```python
from build123d import *

# Parameters (mm, degrees)
CUT_EXTRUDE_1_DEPTH = 125.373429638


with BuildPart() as part:
    # 草图1 → 旋转1 (revolve)
    with BuildSketch(Plane.XY, mode=Mode.PRIVATE) as revolve_1_sk:
        with BuildLine():
            Line((45, 37.5), (25, 37.5))
            ThreePointArc((25, 37.5), (0, 22.5), (-25, 37.5))
            Line((-25, 37.5), (-45, 37.5))
            ThreePointArc((-45, 37.5), (-71.516504294, 26.516504294), (-82.5, 0))
            Line((-82.5, 0), (82.5, 0))
            ThreePointArc((82.5, 0), (71.516504294, 26.516504294), (45, 37.5))
        make_face()
    revolve(revolve_1_sk.sketch.rotate(Axis((-82.5, 0, 0), (1, 0, 0)), 180), axis=Axis((-82.5, 0, 0), (1, 0, 0)))

    # 草图2 → 切除-拉伸1 (cut, through all)
    with BuildSketch(Plane(origin=(30, 0, 0), x_dir=(0, 0, -1), z_dir=(1, 0, 0))):
        with BuildLine():
            Line((10, 36.142080737), (10, 10))
            Line((10, 10), (36.142080737, 10))
            ThreePointArc((36.142080737, 10), (26.516504294, 26.516504294), (10, 36.142080737))
        make_face()
        with BuildLine():
            Line((-10, 10), (-36.142080737, 10))
            ThreePointArc((-36.142080737, 10), (-26.516504294, 26.516504294), (-10, 36.142080737))
            Line((-10, 36.142080737), (-10, 10))
        make_face()
        with BuildLine():
            Line((-10, -10), (-36.142080737, -10))
            ThreePointArc((-36.142080737, -10), (-26.516504294, -26.516504294), (-10, -36.142080737))
            Line((-10, -36.142080737), (-10, -10))
        make_face()
        with BuildLine():
            Line((10, -10), (36.142080737, -10))
            ThreePointArc((36.142080737, -10), (26.516504294, -26.516504294), (10, -36.142080737))
            Line((10, -36.142080737), (10, -10))
        make_face()
    cut_extrude_1 = extrude(amount=CUT_EXTRUDE_1_DEPTH, mode=Mode.SUBTRACT)

    # 镜向1: 切除-拉伸1 across plane
    add(cut_extrude_1.mirror(Plane(origin=(0, 0, 0), x_dir=(0, 0, 1), z_dir=(1, 0, 0))), mode=Mode.SUBTRACT)


solid = part.part
```
Geometry: final body of the model. Coordinates: model frame, mm. A direction names the side the tool comes from. Coordinates: 2 decimals unless noted, no trailing zeros. Order: outer loops, then holes, each group sorted by start corner. A loop starts at its lowest first (then second) coordinate and runs counter-clockwise, first axis right, second up. Notation, with made-up numbers: (-21.5, -9) -> (-7.5, -9) arc R29 ccw to (-7.5, 17) -> close; hole circle Ø9 at (4.5, 63). An arc over 180 degrees is marked (long way). Write item = value, one per line.
(1) Access query for faces 1 (the flat face through (-49, -10, 23)), 2 (the flat face through (-30, -20, -20)), 3 (the flat face through (30, 20, 20)), 4 (the flat face through (49, -20, -10)). Directions: +Z, -Z, +X, -X, +Y, -Y. A direction counts if a zero-diameter tool reaches every point of the face in a straight line with its end or side. Return the directions, or none.
Solved:
face_1 = +Z, -X, -Y
face_2 = -Z, -X, -Y
face_3 = +Z, +X, +Y
face_4 = -Z, +X, -Y
(2) Cut plane B-B on x = -73. Return loops of the section in (y, z).
Solved:
outline = (-22.85, -10) -> (-10, -10) -> (-10, -22.85) arc R24.94 ccw to (10, -22.85) -> (10, -10) -> (22.85, -10) arc R24.94 ccw to (22.85, 10) -> (10, 10) -> (10, 22.85) arc R24.94 ccw to (-10, 22.85) -> (-10, 10) -> (-22.85, 10) arc R24.94 ccw to start
(3) Cut plane D-D on x = -34. Return loops of the section in (y, z).
Solved:
outline = (-36.14, -10) -> (-10, -10) -> (-10, -36.14) arc R37.5 ccw to (10, -36.14) -> (10, -10) -> (36.14, -10) arc R37.5 ccw to (36.14, 10) -> (10, 10) -> (10, 36.14) arc R37.5 ccw to (-10, 36.14) -> (-10, 10) -> (-36.14, 10) arc R37.5 ccw to start
(4) Cut plane A-A on z = 0. Return loops of the section in (x, y).
Solved:
outline = (-45, -37.5) -> (-25, -37.5) arc R28.33 cw to (25, -37.5) -> (45, -37.5) arc R37.5 ccw to (45, 37.5) -> (25, 37.5) arc R28.33 cw to (-25, 37.5) -> (-45, 37.5) arc R37.5 ccw to start
(5) Pin query (flat end, axial travel): pin 1 Ø6 at (x, y) = (17, 25) entering from -Z; pin 2 Ø6 at (x, z) = (-36.5, -10.5) entering from -Y; pin 3 Ø2 at (y, z) = (-22.5, -19) entering from -X. Return the tip coordinate at first contact, or that it passes through.
Solved:
pin_1 = -19.31
pin_2 = -36.74
pin_3 = -30
(6) Line query: line 1 (Y direction, x = -64, z = -29.5); line 2 (X direction, y = 16, z = 31). Output: solid intervals per line, ascending.
Solved:
line_1 = -10 to 10
line_2 = -30 to -23.42, 23.42 to 30
